Autodesk Inventor part; units mm, degrees
ref_plane "YZ Plane" through (0, 0, 0) normal (1, 0, 0) x (0, 1, 0)
ref_plane "XZ Plane" through (0, 0, 0) normal (0, 1, 0) x (-1, 0, 0)
ref_plane "XY Plane" through (0, 0, 0) normal (0, 0, 1) x (1, 0, 0)
sketch "Sketch1" plane through (0, 0, 0) normal (0, 1, 0) x (-1, 0, 0)
  line L0 (0, 0) -> (130, 0)
  line L1 (130, 0) -> (130, -116.2)
  line L2 (130, -116.2) -> (0, -116.2)
  line L3 (0, -116.2) -> (0, 0)
  dimension "d0" = 130
  dimension "d1" = 116.2
extrude "Extrusion1" add sketch "Sketch1" along normal blind 5
sketch "Sketch2" plane through (0, 5, 0) normal (0, 1, 0) x (1, 0, 0)
  line L0 (-10, -25.3077) -> (-10, 177.8334) construction
  line L1 (0, 0) -> (0, 116.2) construction
  line L2 (-130, 0) -> (0, 0) construction
  line L3 (-47, -19.5328) -> (-47, 162.8865) construction
  line L4 (0, 116.2) -> (-130, 116.2) construction
  point P0 (-10, 16.7)
  point P1 (-10, 66.7)
  point P2 (-47, 111.7)
  point P3 (-47, 43.95)
  point P4 (-47, 17.95)
  dimension "d4" = 10
  dimension "d5" = 16.7
  dimension "d6" = 50
  dimension "d7" = 47
  dimension "d8" = 4.5
  dimension "d9" = 72.25
  dimension "d10" = 98.25
hole "Hole1" at (-10, 5, -16.7) at (-10, 5, -66.7) direction (0, -1, 0) diameter 3.8 end through all
sketch "Sketch3" plane through (0, 5, 0) normal (0, 1, 0) x (1, 0, 0)
  line L0 (-105, 0) -> (-25, 0)
  line L1 (-25, 0) -> (-25, 8)
  line L2 (-27, 10) -> (-103, 10)
  line L3 (-105, 8) -> (-105, 0)
  line L4 (-130, 116.2) -> (-130, 0)
  line L5 (0, 0) -> (0, 116.2)
  arc A0 (-103, 10) -> (-105, 8) centre (-103, 8) ccw
  arc A1 (-25, 8) -> (-27, 10) centre (-27, 8) ccw
  dimension "d18" = 10
  dimension "d19" = 25
  dimension "d20" = 25
  dimension "d21" = 2
extrude "Extrusion2" cut sketch "Sketch3" against normal blind 5
fillet "Fillet1" radius 2 2 edges at (-105, 2.5, 0) (-25, 2.5, 0)
sketch "Sketch4" plane through (0, 5, 0) normal (0, 1, 0) x (1, 0, 0)
  circle A0 centre (-65.75, 67.1) radius 6
  line L0 (0, 0) -> (0, 116.2)
  line L1 (-23, 0) -> (0, 0)
  dimension "d25" = 12
  dimension "d26" = 65.75
  dimension "d27" = 67.1
extrude "Extrusion3" cut sketch "Sketch4" against normal blind 5
sketch "Sketch5" plane through (0, 5, 0) normal (0, 1, 0) x (1, 0, 0)
  line L0 (-91.5, 130.6682) -> (-91.5, -27.2079) construction
  line L1 (0, 0) -> (0, 116.2) construction
  line L2 (0, 116.2) -> (-130, 116.2) construction
  point P0 (-91.5, 104.2)
  point P1 (-91.5, 73.2)
  dimension "d30" = 91.5
  dimension "d31" = 12
  dimension "d32" = 43
hole "Hole2" at (-91.5, 5, -104.2) at (-91.5, 5, -73.2) direction (0, -1, 0) diameter 3.8 end through all
sketch "Sketch6" plane through (0, 5, 0) normal (0, 1, 0) x (1, 0, 0)
  line L0 (-13, 148.9997) -> (-13, -38.8385) construction
  line L1 (0, 0) -> (0, 116.2)
  line L2 (0, 116.2) -> (-130, 116.2)
  line L3 (-44, 144.1508) -> (-44, -38.8385) construction
  line L4 (-14, 12.9628) -> (-14, -11.5017) construction
  line L5 (-23, 0) -> (0, 0) construction
  point P0 (-13, 80.2)
  point P1 (-13, 32.2)
  point P2 (-44, 70.2)
  point P3 (-44, 32.2)
  point P4 (-14, 6.7)
  dimension "d40" = 13
  dimension "d41" = 36
  dimension "d42" = 84
  dimension "d50" = 44
  dimension "d51" = 46
  dimension "d52" = 84
  dimension "d53" = 14
  dimension "d54" = 6.7
hole "Hole3" at (-13, 5, -80.2) at (-13, 5, -32.2) at (-44, 5, -32.2) at (-44, 5, -70.2) at (-14, 5, -6.7) direction (0, -1, 0) diameter 3.8 end through all
sketch "Sketch7" plane through (-130, 0, -116.2) normal (-1, 0, 0) x (0, 0, 1)
  line L0 (116.2, 0) -> (56.2, 0)
  line L1 (56.2, 0) -> (56.2, 5)
  line L2 (56.2, 5) -> (116.2, 5)
  line L3 (116.2, 5) -> (116.2, 0)
  dimension "d55" = 60
  dimension "d56" = 5
extrude "Extrusion4" add sketch "Sketch7" along normal blind 35
fillet "Fillet2" radius 10 1 edges at (-130, 2.5, -60)
sketch "Sketch8" plane through (0, 5, 0) normal (0, 1, 0) x (1, 0, 0)
  line L0 (-107, 0) -> (-165, 0)
  line L1 (-165, 0) -> (-165, 60)
  point P0 (0, 0)
  point P1 (-157.75, 19.5)
  dimension "d60" = 19.5
  dimension "d61" = 7.25
hole "Hole4" at (-157.75, 5, -19.5) direction (0, -1, 0) diameter 3.8 end through all
sketch "Sketch9" plane through (0, 5, 0) normal (0, 1, 0) x (1, 0, 0)
  line L0 (-24.65, 135.1246) -> (-24.65, 98.3323) construction
  line L1 (0, 0) -> (0, 116.2)
  line L2 (-34.65, 134.2) -> (-14.65, 134.2)
  line L3 (-14.65, 134.2) -> (-14.65, 98.2)
  line L4 (-14.65, 98.2) -> (-34.65, 98.2)
  line L5 (-34.65, 98.2) -> (-34.65, 134.2)
  line L6 (0, 116.2) -> (-130, 116.2)
  line L7 (-34.65, 134.2) -> (-14.65, 98.2) construction
  line L8 (-14.65, 134.2) -> (-34.65, 98.2) construction
  line L9 (-14.65, 106.2) -> (-20.65, 98.2)
  line L10 (-34.65, 106.2) -> (-28.65, 98.2)
  line L11 (-34.65, 116.2) -> (-14.65, 116.2)
  point P0 (-24.65, 116.2)
  dimension "d69" = 24.65
  dimension "d70" = 20
  dimension "d71" = 36
  dimension "d72" = 10
  dimension "d73" = 8
extrude "Extrusion5" cut sketch "Sketch9" against normal through all contours L6 L3 L9 L4 L10 L5
fillet "Fillet3" radius 2 4 edges at (-34.65, 2.5, -106.2) (-28.65, 2.5, -98.2) (-20.65, 2.5, -98.2) (-14.65, 2.5, -106.2)
sketch "Sketch10" plane through (0, 5, 0) normal (0, 1, 0) x (1, 0, 0)
  line L0 (-34.65, 106.8667) -> (-34.65, 116.2)
  line L1 (-34.65, 116.2) -> (-130, 116.2)
  line L2 (-130, 116.2) -> (-130, 70)
  arc A0 (-140, 60) -> (-130, 70) centre (-140, 70) ccw
  line L3 (-140, 60) -> (-165, 60)
  line L4 (-165, 0) -> (-165, 60)
  line L5 (-107, 0) -> (-165, 0)
  arc A1 (-107, 0) -> (-105, 2) centre (-107, 2) ccw
  line L6 (-105, 2) -> (-105, 8)
  arc A2 (-103, 10) -> (-105, 8) centre (-103, 8) ccw
  line L7 (-103, 10) -> (-27, 10)
  arc A3 (-25, 8) -> (-27, 10) centre (-27, 8) ccw
  line L8 (-25, 8) -> (-25, 2)
  arc A4 (-25, 2) -> (-23, 0) centre (-23, 2) ccw
  line L9 (-23, 0) -> (0, 0)
  line L10 (0, 0) -> (0, 116.2)
  line L11 (0, 116.2) -> (-14.65, 116.2)
  line L12 (-14.65, 116.2) -> (-14.65, 106.8667)
  arc A5 (-15.05, 105.6667) -> (-14.65, 106.8667) centre (-16.65, 106.8667) ccw
  line L13 (-15.05, 105.6667) -> (-20.05, 99)
  arc A6 (-21.65, 98.2) -> (-20.05, 99) centre (-21.65, 100.2) ccw
  line L14 (-21.65, 98.2) -> (-27.65, 98.2)
  arc A7 (-29.25, 99) -> (-27.65, 98.2) centre (-27.65, 100.2) ccw
  line L15 (-29.25, 99) -> (-34.25, 105.6667)
  arc A8 (-34.65, 106.8667) -> (-34.25, 105.6667) centre (-32.65, 106.8667) ccw
  circle A9 centre (-157.75, 19.5) radius 1.9
  circle A10 centre (-44, 70.2) radius 1.9
  circle A11 centre (-13, 32.2) radius 1.9
  circle A12 centre (-13, 80.2) radius 1.9
  circle A13 centre (-44, 32.2) radius 1.9
  circle A14 centre (-14, 6.7) radius 1.9
  circle A15 centre (-91.5, 104.2) radius 1.9
  circle A16 centre (-91.5, 73.2) radius 1.9
  circle A17 centre (-65.75, 67.1) radius 6
  circle A18 centre (-10, 16.7) radius 1.9
  circle A19 centre (-10, 66.7) radius 1.9
  line L16 (-65.75, 187.4389) -> (-65.75, -19.4667) construction
  line L17 (-34.65, 116.2) -> (-130, 116.2)
  circle A20 centre (-65.75, 67.1) radius 6
  line L18 (-69.75, 116.2) -> (-61.75, 116.2)
  line L19 (-61.75, 116.2) -> (-61.75, 71.5721)
  line L20 (-61.75, 71.5721) -> (-69.75, 71.5721)
  line L21 (-69.75, 71.5721) -> (-69.75, 116.2)
  dimension "d77" = 8
extrude "Extrusion6" cut sketch "Sketch10" against normal through all contours L19 A17 L21 L1
fillet "Fillet4" radius 2 4 edges at (-69.75, 2.5, -116.2) (-61.75, 2.5, -116.2) (-69.75, 2.5, -71.5721) (-61.75, 2.5, -71.5721)
sketch "Sketch11" plane through (0, 5, 0) normal (0, 1, 0) x (1, 0, 0)
  line L0 (-75.5, 139.1066) -> (-75.5, -104.8745) construction
  line L1 (0, 0) -> (0, 116.2) construction
  line L2 (-71.75, 116.2) -> (-130, 116.2) construction
  point P0 (-75.5, 31.2)
  point P1 (-75.5, 81.2)
  dimension "d81" = 75.5
  dimension "d82" = 35
  dimension "d83" = 85
hole "Hole5" at (-75.5, 5, -31.2) at (-75.5, 5, -81.2) direction (0, -1, 0) diameter 3.8 end through all
properties part number "Bottle side plate"
Geometry check sheet. Reference: the model listing, model coordinates, mm. A direction names the side the tool comes from. Give positions to 0.01 mm unless a question says otherwise; leave off trailing zeros. Loops run counter-clockwise (first coordinate to the right, second up) from the corner with the lowest first, then second, coordinate; pieces in that order, holes last.
(1) Thickness scan on L1, parallel to X at y = 2.45, z = -73; L2, parallel to Z at x = -44, y = 2.35; L3, parallel to X at y = 3.1, z = -100. Record the ranges inside material, lowest first.
From the geometry:
L1: x = -130 to -93.39, -89.61 to -69.75, -61.75 to 0
L2: z = -116.2 to -72.1, -68.3 to -34.1, -30.3 to -10
L3: x = -130 to -69.75, -61.75 to -30, -19.3 to 0
(2) Section check A-A on x = -91.5. Record the cut outline in (y, z).
From the geometry:
outline: (0, -116.2) - (5, -116.2) - (5, -106.1) - (0, -106.1) - close; (0, -102.3) - (5, -102.3) - (5, -75.1) - (0, -75.1) - close; (0, -71.3) - (5, -71.3) - (5, -10) - (0, -10) - close
(3) Section check C-C on x = -153. Record the cut outline in (y, z), then the cut area to 3 significant figures.
From the geometry:
outline: (0, -60) - (5, -60) - (5, 0) - (0, 0) - close
area: 300 mm2
(4) Depth check by flat-ended pin: pin 1 Ø2.5 at (x, y) = (-153, 2.5) entering from -Z; pin 2 Ø3 at (y, z) = (3, -89.5) entering from -X. Enter the tip coordinate at first touch or a pass-through.
From the geometry:
pin 1: stops at z = -60
pin 2: stops at x = -130
(5) Set-up check for faces 1 (the flat face through (-152, 2, -60)), 2 (the flat face through (-17.5, 2.5, -102.4)), 3 (the flat face through (-105, 3, -5)): record each of +Z, -Z, +X, -X, +Y, -Y from which the full face is reachable in a straight line by a thin tool's end or side.
From the geometry:
face 1: -Z, -X, +Y, -Y
face 2: -Z, +Y, -Y
face 3: +Z, +Y, -Y
(6) Release check for a two-part mould opening along Z. For faces 4 (the flat face through (-25, 3, -5)), 5 (the flat face through (-25, 3, -98.2)), 6 (the cylindrical face through (-155.895, 2.465, -19.912)) record: released by +Z, released by -Z, zero draft, split by the parting line, or undercut.
From the geometry:
face 4: zero draft
face 5: released by -Z
face 6: undercut
(7) Section check B-B on y = 3.8. Count the separate pieces of the cut face and the enclosed holes in it, then the cut area to 3 significant figures.
From the geometry:
separate pieces: 1
enclosed holes: 12
area: 15,500 mm2
